Part model, mm, in its own coordinate system. A direction names the side the tool comes from. Round coordinates to 2 decimals unless told otherwise and drop trailing zeros. Loops run counter-clockwise (first coordinate to the right, second up) from the corner with the lowest first, then second, coordinate; pieces in that order, holes last.
from build123d import *

# Parameters (mm, degrees)
EXTRUDE_1_DEPTH     = 10
SKETCH_2_R          = 1.75
CUT_EXTRUDE_1_DEPTH = 10


with BuildPart() as part:
    # 草图1 → 凸台-拉伸1 (new body)
    with BuildSketch(Plane(origin=(0, 0, 0), x_dir=(1, 0, 0), z_dir=(0, 1, 0))):
        with BuildLine():
            Line((6.15, 0), (6.15, -1.65))
            Line((6.15, -1.65), (11.15, -1.65))
            Line((11.15, -1.65), (11.15, -3.65))
            Line((11.15, -3.65), (6.15, -3.65))
            Line((6.15, -3.65), (2.65, -3.65))
            Line((2.65, -3.65), (2.65, -2.65))
            Line((2.65, -2.65), (2.65, 0))
            ThreePointArc((2.65, 0), (0, 2.65), (-2.65, 0))
            Line((-2.65, 0), (-2.65, -2.65))
            Line((-2.65, -2.65), (-2.65, -3.65))
            Line((-2.65, -3.65), (-6.15, -3.65))
            Line((-6.15, -3.65), (-11.15, -3.65))
            Line((-11.15, -3.65), (-11.15, -1.65))
            Line((-11.15, -1.65), (-6.15, -1.65))
            Line((-6.15, -1.65), (-6.15, 0))
            ThreePointArc((-6.15, 0), (0, 6.15), (6.15, 0))
        make_face()
    extrude(amount=EXTRUDE_1_DEPTH)

    # 草图2 → 切除-拉伸1 (cut)
    with BuildSketch(Plane(origin=(0, 0, 1.65), x_dir=(-1, 0, 0), z_dir=(0, 0, -1))):
        with Locations((8.65, 5)):
            Circle(SKETCH_2_R)
        with Locations(Location((-8.65, 5, 0), (0, 0, 180))):
            Circle(SKETCH_2_R)
    extrude(amount=-CUT_EXTRUDE_1_DEPTH, mode=Mode.SUBTRACT)


solid = part.part
1) Slice it at B-B, the plane z = 2.25. Give the cut face in (x, y).
Values:
outline: (-11.15, 0) - (-2.65, 0) - (-2.65, 10) - (-11.15, 10) - close; (2.65, 0) - (11.15, 0) - (11.15, 10) - (2.65, 10) - close; hole circle Ø3.5 at (-8.65, 5); hole circle Ø3.5 at (8.65, 5)
2) Slice it at D-D, the plane x = 8.5. Give the cut face in (y, z).
Values:
outline: (0, 1.65) - (3.26, 1.65) - (3.26, 3.65) - (0, 3.65) - close; (6.74, 1.65) - (10, 1.65) - (10, 3.65) - (6.74, 3.65) - close
3) Slice it at C-C, the plane z = 1. Give the cut face in (x, y).
Values:
outline: (-6.15, 0) - (-2.65, 0) - (-2.65, 10) - (-6.15, 10) - close; (2.65, 0) - (6.15, 0) - (6.15, 10) - (2.65, 10) - close
4) Slice it at A-A, the plane y = 5. Give the cut face in (x, z), then the cut area to 3 significant figures.
Values:
outline: (-11.15, 1.65) - (-10.4, 1.65) - (-10.4, 3.65) - (-11.15, 3.65) - close; (-6.9, 1.65) - (-6.15, 1.65) - (-6.15, 0) arc R6.15 ccw to (6.15, 0) - (6.15, 1.65) - (6.9, 1.65) - (6.9, 3.65) - (2.65, 3.65) - (2.65, 0) arc R2.65 cw to (-2.65, 0) - (-2.65, 3.65) - (-6.9, 3.65) - close; (10.4, 1.65) - (11.15, 1.65) - (11.15, 3.65) - (10.4, 3.65) - close
area: 79.9 mm2
5) Drop flat-ended pins along their axis: pin 1 Ø5.5 at (x, y) = (-9, 6.5) entering from -Z; pin 2 Ø0.5 at (y, z) = (7.5, 0.5) entering from -X; pin 3 Ø1 at (y, z) = (4.5, -4) entering from -X. Give the stop position or say it passes through.
Values:
pin 1: stops at z = 1.65
pin 2: stops at x = -6.15
pin 3: stops at x = -5.06
6) Wall check: line 1 along Y through (x, z) = (-8.65, 2.9); line 2 along X through (y, z) = (6.5, 1.75); line 3 along X through (y, z) = (9, 1). Give the ranges that are in metal, low to high.
Values:
line 1: y = 0 to 3.25, 6.75 to 10
line 2: x = -11.15 to -9.55, -7.75 to -2.65, 2.65 to 7.75, 9.55 to 11.15
line 3: x = -6.15 to -2.65, 2.65 to 6.15
7) Mould opens along Y. For faces 6 (the face through (3, 0, -1)), 7 (the face through (6.15, 5, 1)), 8 (the face through (-9.46, 3.45, 2.64)) say: released by +Y, released by -Y, zero draft, split by the parting line, or undercut.
Values:
face 6: released by -Y
face 7: zero draft
face 8: undercut
8) Tool access for faces 1 (the face through (6, 5, 3.65)), 2 (the face through (3, 10, -1)), 3 (the face through (-2.65, 5, 2)), 4 (the face through (-10.4, 3.8, 1.65)), 5 (the face through (7, 4, 1.65)): list every direction of +Z, -Z, +X, -X, +Y, -Y with a clear straight run to the whole face (end or side of a thin tool).
Values:
face 1: +Z, +X, -X, +Y, -Y
face 2: +Z, -Z, +X, -X, +Y
face 3: +Z, +Y, -Y
face 4: -Z, -X, +Y, -Y
face 5: -Z, +X, +Y, -Y
